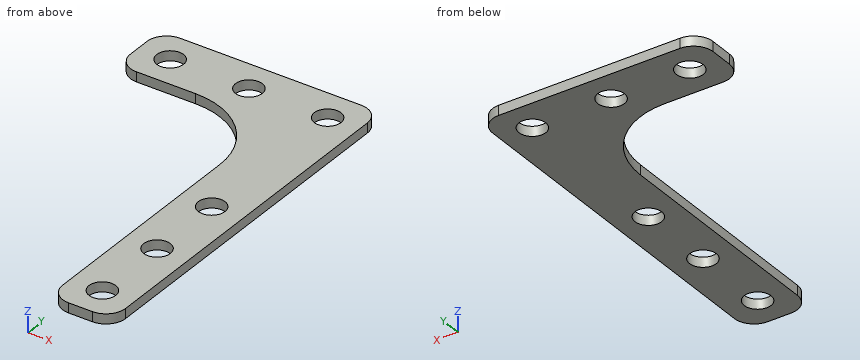
Autodesk Inventor part; units mm, degrees
ref_plane "YZ Plane" through (0, 0, 0) normal (1, 0, 0) x (0, 1, 0)
ref_plane "XZ Plane" through (0, 0, 0) normal (0, 1, 0) x (-1, 0, 0)
ref_plane "XY Plane" through (0, 0, 0) normal (0, 0, 1) x (1, 0, 0)
sketch "Sketch1" plane through (0, 0, 0) normal (0, 0, 1) x (1, 0, 0)
  circle A0 centre (0, 0) radius 2.159
  line L0 (0, 0) -> (-38.1, 0) construction
  line L1 (0, 0) -> (0, -26.9418) construction
  circle A1 centre (-12.7, 0) radius 2.159
  circle A2 centre (-25.4, 0) radius 2.159
  circle A3 centre (0, -26.9418) radius 2.159
  circle A4 centre (0, -39.6418) radius 2.159
  circle A5 centre (0, -52.3418) radius 2.159
  line L2 (5.08, -57.4218) -> (-5.08, -57.4218)
  line L3 (-5.08, -57.4218) -> (-5.08, 5.08)
  line L4 (-5.08, 5.08) -> (5.08, 5.08)
  line L5 (5.08, 5.08) -> (5.08, -57.4218)
  circle A6 centre (0, -52.3418) radius 5.08 construction
  circle A7 centre (0, 0) radius 5.08 construction
  line L6 (5.08, 5.08) -> (-30.48, 5.08)
  line L7 (-30.48, 5.08) -> (-30.48, -5.08)
  line L8 (-30.48, -5.08) -> (5.08, -5.08)
  line L9 (5.08, -5.08) -> (5.08, 5.08)
  circle A8 centre (-25.4, 0) radius 5.08 construction
  point P0 (-5.08, 5.08)
  point P1 (-5.08, -5.08)
  point P2 (-5.08, 5.08)
  point P3 (5.08, -5.08)
  dimension "d5" = 12.7
  dimension "d21" = 26.9418
  dimension "d22" = 4.318
  dimension "d25" = 12.7
  dimension "d30" = 10.16
extrude "Extrusion1" add sketch "Sketch1" along normal blind 1.5875
fillet "Fillet1" radius 3.175 5 edges at (-30.48, -5.08, 0.7937) (-30.48, 5.08, 0.7937) (5.08, 5.08, 0.7937) (5.08, -57.4218, 0.7937) (-5.08, -57.4218, 0.7937)
fillet "Fillet2" radius 12.7 1 edges at (-5.08, -5.08, 0.7937)
properties part number "Inner_Strut_Gusset" material "Aluminum 6061"
Read the model definition and answer for the solid it produces. Units are mm, in the model's axes. Give positions to 0.01 mm unless a question says otherwise; leave off trailing zeros. Loops run counter-clockwise (first coordinate to the right, second up) from the corner with the lowest first, then second, coordinate; pieces in that order, holes last. Notation, with made-up numbers: (-37, -4.5) -> (21, -4.5) arc R14 ccw to (21, -0.5) -> close; hole circle Ø11 at (-19.5, 24). An arc over 180 degrees is marked (long way). Use a Markdown table: item, result.
Q1. Find the intervals of material crossed by line 1 along Y through (x, z) = (0, 0.65); line 2 along Y through (x, z) = (-25.4, 0.3); line 3 along Y through (x, z) = (-0.5, 1.45), in increasing order.
Solved:
| item | result |
|---|---|
| line 1 | y = -57.42 to -54.5, -50.18 to -41.8, -37.48 to -29.1, -24.78 to -2.16, 2.16 to 5.08 |
| line 2 | y = -5.08 to -2.16, 2.16 to 5.08 |
| line 3 | y = -57.42 to -54.44, -50.24 to -41.74, -37.54 to -29.04, -24.84 to -2.1, 2.1 to 5.08 |
Q2. Section D-D, the plane z = 0.6 is taken. Determine the outline of the cut face in (x, y) (3 decimals), then the cut area to 3 significant figures.
Solved:
| item | result |
|---|---|
| outline | (-30.48, -1.905) arc R3.175 ccw to (-27.305, -5.08) -> (-17.78, -5.08) arc R12.7 cw to (-5.08, -17.78) -> (-5.08, -54.247) arc R3.175 ccw to (-1.905, -57.422) -> (1.905, -57.422) arc R3.175 ccw to (5.08, -54.247) -> (5.08, 1.905) arc R3.175 ccw to (1.905, 5.08) -> (-27.305, 5.08) arc R3.175 ccw to (-30.48, 1.905) -> close; hole circle Ø4.318 at (-25.4, 0); hole circle Ø4.318 at (-12.7, 0); hole circle Ø4.318 at (0, -52.342); hole circle Ø4.318 at (0, -39.642); hole circle Ø4.318 at (0, -26.942); hole circle Ø4.318 at (0, 0) |
| area | 829 mm^2 |
Q3. Section C-C, the plane x = 0 is taken. Determine the outline of the cut face in (y, z), then the cut area to 3 significant figures.
Solved:
| item | result |
|---|---|
| outline | (-57.42, 0) -> (-54.5, 0) -> (-54.5, 1.59) -> (-57.42, 1.59) -> close; (-50.18, 0) -> (-41.8, 0) -> (-41.8, 1.59) -> (-50.18, 1.59) -> close; (-37.48, 0) -> (-29.1, 0) -> (-29.1, 1.59) -> (-37.48, 1.59) -> close; (-24.78, 0) -> (-2.16, 0) -> (-2.16, 1.59) -> (-24.78, 1.59) -> close; (2.16, 0) -> (5.08, 0) -> (5.08, 1.59) -> (2.16, 1.59) -> close |
| area | 71.8 mm^2 |
Q4. Section A-A, the plane x = -25.4 is taken. Determine the outline of the cut face in (y, z), then the cut area to 3 significant figures.
Solved:
| item | result |
|---|---|
| outline | (-5.08, 0) -> (-2.16, 0) -> (-2.16, 1.59) -> (-5.08, 1.59) -> close; (2.16, 0) -> (5.08, 0) -> (5.08, 1.59) -> (2.16, 1.59) -> close |
| area | 9.27 mm^2 |
Q5. Section B-B, the plane y = 0 is taken. Determine the outline of the cut face in (x, z), then the cut area to 3 significant figures.
Solved:
| item | result |
|---|---|
| outline | (-30.48, 0) -> (-27.56, 0) -> (-27.56, 1.59) -> (-30.48, 1.59) -> close; (-23.24, 0) -> (-14.86, 0) -> (-14.86, 1.59) -> (-23.24, 1.59) -> close; (-10.54, 0) -> (-2.16, 0) -> (-2.16, 1.59) -> (-10.54, 1.59) -> close; (2.16, 0) -> (5.08, 0) -> (5.08, 1.59) -> (2.16, 1.59) -> close |
| area | 35.9 mm^2 |
Q6. This flat-tipped pin is pushed along its axis until it touches: pin 1 (7 mm diameter, centred on x = 0, y = -39.64, fed in from +Z). Where does it stop, or does it pass through?
Solved:
| item | result |
|---|---|
| pin 1 | stops at z = 1.59 |
